```python
from build123d import *

# Parameters (mm, degrees)
SKETCH1_R           = 82.5
BOSS_EXTRUDE1_DEPTH = 3
SKETCH2_R           = 1.75
SKETCH2_R_2         = 22
CUT_EXTRUDE1_DEPTH  = 3
SKETCH3_R           = 1.75
CUT_EXTRUDE2_DEPTH  = 117.711181984
CIRPATTERN1_COUNT   = 12
CUT_EXTRUDE3_DEPTH  = 3


with BuildPart() as part:
    # Sketch1 → Boss-Extrude1 (new body)
    with BuildSketch(Plane(origin=(0, 0, 0), x_dir=(1, 0, 0), z_dir=(0, 1, 0))):
        with Locations(Location((0, 0, 0), (0, 0, 270))):
            Circle(SKETCH1_R)
    extrude(amount=BOSS_EXTRUDE1_DEPTH)

    # Sketch2 → Cut-Extrude1 (cut)
    with BuildSketch(Plane(origin=(0, 3, 0), x_dir=(1, 0, 0), z_dir=(0, 1, 0))):
        with Locations(Location((57, 0, 0), (0, 0, 270))):
            Circle(SKETCH2_R)
        with Locations(Location((0, 0, 0), (0, 0, 270))):
            Circle(SKETCH2_R_2)
        with Locations(Location((-57, 0, 0), (0, 0, 270))):
            Circle(SKETCH2_R)
    extrude(amount=-CUT_EXTRUDE1_DEPTH, mode=Mode.SUBTRACT)

    # Sketch3 → Cut-Extrude2 (cut, through all)
    with BuildSketch(Plane(origin=(0, 3, 0), x_dir=(1, 0, 0), z_dir=(0, 1, 0))):
        with Locations(Location((72.444436972, -19.411428383, 0), (0, 0, 270))):
            Circle(SKETCH3_R)
    cut_extrude2 = extrude(amount=-CUT_EXTRUDE2_DEPTH, mode=Mode.SUBTRACT)

    # CirPattern1: Cut-Extrude2 ×12 about axis
    cirpattern1_axis = Axis((0, 0, 0), (0, 1, 0))
    for i in range(1, CIRPATTERN1_COUNT):
        add(cut_extrude2.rotate(cirpattern1_axis, i * 360 / CIRPATTERN1_COUNT), mode=Mode.SUBTRACT)

    # Sketch4 → Cut-Extrude3 (cut)
    with BuildSketch(Plane(origin=(0, 3, 0), x_dir=(1, 0, 0), z_dir=(0, 1, 0))):
        with BuildLine():
            Line((0, 67.5), (-15, 67.5))
            Line((-15, 67.5), (-15, 37.5))
            Line((-15, 37.5), (0, 37.5))
            Line((0, 37.5), (0, 22))
            ThreePointArc((0, 22), (22, 0), (0, -22))
            Line((0, -22), (0, -37.5))
            Line((0, -37.5), (15, -37.5))
            Line((15, -37.5), (15, -67.5))
            Line((15, -67.5), (0, -67.5))
            Line((0, -67.5), (0, -82.5))
            ThreePointArc((0, -82.5), (82.5, 0), (0, 82.5))
            Line((0, 82.5), (0, 67.5))
        make_face()
    extrude(amount=-CUT_EXTRUDE3_DEPTH, mode=Mode.SUBTRACT)


solid = part.part
```
Model file for the job. Use its own axes, mm. A direction names the side the tool comes from. Give positions to 0.01 mm unless a question says otherwise; leave off trailing zeros. Write each loop counter-clockwise with the first axis right and the second up, starting at its lowest first coordinate (ties: lowest second). Pieces come first, ordered by that corner, then holes. Notation, with made-up numbers: M 77,8.25 L 102,8.25 A12 cw 102,28.25 Z; hole C 52.5,6.25 d10. An arc over 180 degrees is marked long. Use a Markdown table: item, result.
1) Pull direction Z, two halves, no side cores. Call faces 5 (the flat face through (7, 2, 37.5)), 6 (the cylindrical face through (-82.48, 1.48, -1.81)), 7 (the flat face through (0, 2, 75)), 8 (the cylindrical face through (-70.736, 1.521, -19.032)): +Z half, -Z half, draft (parallel to the pull), parting line (faces both ways), or undercut.
Responses:
| item | result |
|---|---|
| face 5 | -Z half |
| face 6 | parting line |
| face 7 | draft |
| face 8 | undercut |
2) Cut at C-C (y = 0.5). List the corners of the cut face in (x, z), and give its area (3 significant figures).
Responses:
| item | result |
|---|---|
| outline | M -15,-67.5 L -15,-37.5 L 0,-37.5 L 0,-22 A22 cw 0,22 L 0,37.5 L 15,37.5 L 15,67.5 L 0,67.5 L 0,82.5 A82.5 ccw 0,-82.5 L 0,-67.5 Z; hole C -72.44,-19.41 d3.5; hole C -72.44,19.41 d3.5; hole C -57,0 d3.5; hole C -53.03,-53.03 d3.5; hole C -53.03,53.03 d3.5; hole C -19.41,-72.44 d3.5; hole C -19.41,72.44 d3.5 |
| area | 9,860 mm2 |
3) Tool access for faces 1 (the flat face through (8, 2, 67.5)), 2 (the flat face through (0, 2, 30)), 3 (the flat face through (-15, 2, -53)), 4 (the cylindrical face through (-51.7, 1.5, -51.9)): list every direction of +Z, -Z, +X, -X, +Y, -Y with a clear straight run to the whole face (end or side of a thin tool).
Responses:
| item | result |
|---|---|
| face 1 | +Z, +X, +Y, -Y |
| face 2 | -Z, +X, +Y, -Y |
| face 3 | +X, +Y, -Y |
| face 4 | +Y, -Y |
4) Cut at D-D (x = -57). List the corners of the cut face in (y, z), and give its area (3 significant figures).
Responses:
| item | result |
|---|---|
| outline | M 0,-59.64 L 3,-59.64 L 3,-1.75 L 0,-1.75 Z; M 0,1.75 L 3,1.75 L 3,59.64 L 0,59.64 Z |
| area | 347 mm2 |
5) Cut at B-B (x = -8.5). List the corners of the cut face in (y, z), and give its area (3 significant figures).
Responses:
| item | result |
|---|---|
| outline | M 0,-82.06 L 3,-82.06 L 3,-67.5 L 0,-67.5 Z; M 0,-37.5 L 3,-37.5 L 3,-20.29 L 0,-20.29 Z; M 0,20.29 L 3,20.29 L 3,82.06 L 0,82.06 Z |
| area | 281 mm2 |
6) Drill centre lines: line 1 (Z direction, x = -18.5, y = 0.3); line 2 (X direction, y = 2.25, z = 0); line 3 (Z direction, x = -71, y = 2.05). Where is each one in solid material? Low to high. Write a range as from..to.
Responses:
| item | result |
|---|---|
| line 1 | z = -80.4..-73.94, -70.95..-11.91, 11.91..70.95, 73.94..80.4 |
| line 2 | x = -82.5..-58.75, -55.25..-22 |
| line 3 | z = -42.01..-20.4, -18.42..18.42, 20.4..42.01 |
7) Cut at A-A (z = 0). List the corners of the cut face in (x, y).
Responses:
| item | result |
|---|---|
| outline | M -82.5,0 L -58.75,0 L -58.75,3 L -82.5,3 Z; M -55.25,0 L -22,0 L -22,3 L -55.25,3 Z |
8) Pin check, flat tips, straight feed: pin 1 (1.5 mm diameter, centred on x = -38.5, y = 2.5, fed in from -Z); pin 2 (1.5 mm diameter, centred on x = -72.5, z = 19, fed in from -Y); pin 3 (0.9 mm diameter, centred on y = 2, z = -50.5, fed in from +X); pin 4 (1.5 mm diameter, centred on y = 2, z = -30, fed in from +X). Stop position of each tip, or through.
Responses:
| item | result |
|---|---|
| pin 1 | stops at z = -73.36 |
| pin 2 | passes through |
| pin 3 | stops at x = -15 |
| pin 4 | stops at x = 0 |
